from build123d import *

# Parameters (mm, degrees)
SKETCH3_R               = 2.5
CUT_EXTRUDE2_DEPTH      = 13.5
CUT_EXTRUDE2_DEPTH_BACK = 13.5
SKETCH2_R               = 6
CUT_EXTRUDE3_DEPTH      = 183
SKETCH4_R               = 12.5
BOSS_EXTRUDE1_DEPTH     = 35
SKETCH5_R               = 12.5
BOSS_EXTRUDE2_DEPTH     = 35


with BuildPart() as part:
    # Sketch1 → Revolve1 (revolve)
    with BuildSketch(Plane.XY):
        Polygon((0, 0), (0, 3), (10, 3), (10, 12.5), (225, 12.5), (225, 0), align=None)
    revolve(axis=Axis((0, 0, 0), (1, 0, 0)))

    # Sketch3 → Cut-Extrude2 (cut, two sides)
    with BuildSketch(Plane.XY) as cut_extrude2_sk:
        with Locations((5, 0)):
            Circle(SKETCH3_R)
    extrude(amount=CUT_EXTRUDE2_DEPTH, mode=Mode.SUBTRACT)
    extrude(cut_extrude2_sk.sketch, amount=-CUT_EXTRUDE2_DEPTH_BACK, mode=Mode.SUBTRACT)

    # Sketch2 → Cut-Extrude3 (cut)
    with BuildSketch(Plane(origin=(225, 0, 0), x_dir=(0, 0, -1), z_dir=(1, 0, 0))):
        Circle(SKETCH2_R)
    extrude(amount=-CUT_EXTRUDE3_DEPTH, mode=Mode.SUBTRACT)

    # Sketch4 → Boss-Extrude1 (add)
    with BuildSketch(Plane.ZY.offset(-10)):
        with BuildLine():
            Line((-13, 0), (-13, -26))
            ThreePointArc((-13, -26), (0, -39), (13, -26))
            Line((13, -26), (13, 0))
            ThreePointArc((13, 0), (0, 13), (-13, 0))
        make_face()
        Circle(SKETCH4_R, mode=Mode.SUBTRACT)
    extrude(amount=-BOSS_EXTRUDE1_DEPTH)

    # Sketch5 → Boss-Extrude2 (add)
    with BuildSketch(Plane(origin=(45, 0, 0), x_dir=(0, 0, -1), z_dir=(1, 0, 0))):
        with Locations((0, -26)):
            Circle(SKETCH5_R)
    extrude(amount=BOSS_EXTRUDE2_DEPTH)


solid = part.part
Work out the finished part from the listing and answer in its coordinate system (mm). A direction names the side the tool comes from. Round coordinates to 2 decimals unless told otherwise and drop trailing zeros. Loops run counter-clockwise (first coordinate to the right, second up) from the corner with the lowest first, then second, coordinate; pieces in that order, holes last. Notation, with made-up numbers: M 6,61 L 52,61 A31 ccw 52,91 Z; hole C -15,19 d1. An arc over 180 degrees is marked long. One line per question, with ' | ' between items. Start each with the question number.
(1) Flat-ended cylindrical pins translate along their axes: pin 1 Ø13 at (y, z) = (-24, 2) entering from -X; pin 2 Ø7 at (y, z) = (0, 0) entering from +X; pin 3 Ø8 at (y, z) = (-20, 1) entering from +X; pin 4 Ø3 at (x, y) = (5, 0) entering from +Z. Find the tip coordinate at first contact, or state that the pin passes through.
(2) For a pull along Y with two mould halves and no side action, classify faces 1 (the face through (0, 0, 0)), 2 (the face through (62.255, -38.203, 2.71)), 3 (the face through (27, -39, 0)), 4 (the face through (45, -13, 0)) as released by +Y, released by -Y, zero draft, split by the parting line, or undercut.
(3) A cutting plane is placed at B-B on z = 0. Write down the section's boundary in (x, y).
(4) Find the intervals of material crossed by line 1 (Y direction, x = 125, z = 0); line 2 (Y direction, x = 5, z = -0.5); line 3 (X direction, y = 0, z = 0.5), in increasing order.
(5) A cutting plane is placed at A-A on y = -10. Write down the section's boundary in (x, z).
(6) A cutting plane is placed at C-C on x = 71.5. Write down the section's boundary in (y, z), plus the area to 3 significant figures.
(7) A cutting plane is placed at D-D on x = 132. Write down the section's boundary in (y, z), plus the area to 3 significant figures.
(8) A tool of negligible diameter and unlimited length cuts with its end or side. For faces 5 (the face through (136.26, 11.923, 3.755)), 6 (the face through (5.07, 2.77, -1.15)), 7 (the face through (80, -26, 0)), from which of +Z, -Z, +X, -X, +Y, -Y can it reach the whole face along a straight path? Write none if from no direction.
Geometry check:
1) pin 1: stops at x = 10 | pin 2: stops at x = 42 | pin 3: stops at x = 80 | pin 4: passes through
2) face 1: zero draft | face 2: undercut | face 3: released by -Y | face 4: undercut
3) outline: M 0,-3 L 10,-3 L 10,-39 L 45,-39 L 45,-38.5 L 80,-38.5 L 80,-13.5 L 45,-13.5 L 45,-12.5 L 225,-12.5 L 225,-6 L 42,-6 L 42,6 L 225,6 L 225,12.5 L 45,12.5 L 45,13 L 10,13 L 10,3 L 0,3 Z; hole C 5,0 d5
4) line 1: y = -12.5 to -6, 6 to 12.5 | line 2: y = -2.96 to -2.5, 2.5 to 2.96 | line 3: x = 0 to 2.5, 7.5 to 42
5) outline: M 10,-13 L 45,-13 L 45,-7.5 L 225,-7.5 L 225,7.5 L 45,7.5 L 45,13 L 10,13 Z
6) outline: C -26,0 d25; C 0,0 d25; hole C 0,0 d12 | area: 869 mm²
7) outline: C 0,0 d25; hole C 0,0 d12 | area: 378 mm²
8) face 5: +X | face 6: -X | face 7: +Z, -Z, +X, -Y
